Source: CAD feature listing. Evaluate the final solid. Frame: model axes, mm. Coordinates: 2 decimals unless noted, no trailing zeros. Write each loop counter-clockwise with the first axis right and the second up, starting at its lowest first coordinate (ties: lowest second). Pieces come first, ordered by that corner, then holes. Notation, with made-up numbers: (88, 87.25) -> (135, 87.25) arc R23 ccw to (135, 112.25) -> close; hole circle Ø4 at (65, -29.75). An arc over 180 degrees is marked (long way). Write item = value, one per line.
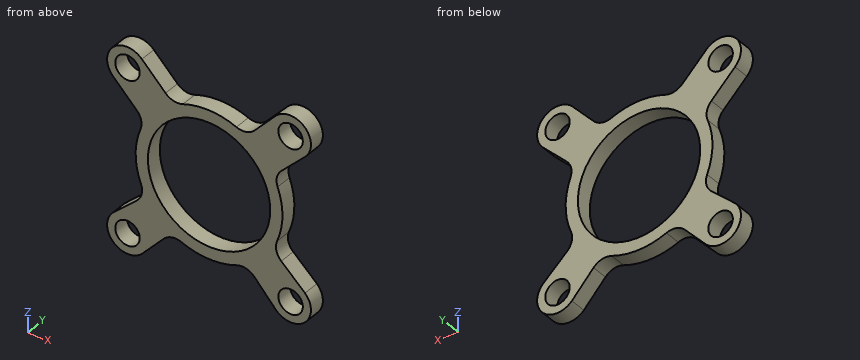
from build123d import *

# Parameters (mm, degrees)
SKETCH1_R           = 7.5
SKETCH1_R_2         = 1.5
BOSS_EXTRUDE1_DEPTH = 2
FILLET1_R           = 2


with BuildPart() as part:
    # Sketch1 → Boss-Extrude1 (new body)
    with BuildSketch(Plane(origin=(0, 0, 0), x_dir=(1, 0, 0), z_dir=(0, 1, 0))):
        with BuildLine():
            Line((-11.767766953, -8.232233047), (-7.881276583, -4.345742677))
            ThreePointArc((-7.881276583, -4.345742677), (-8.999066908, 0.129594703), (-7.75286903, 4.570888514))
            Line((-7.75286903, 4.570888514), (-11.767766953, 8.232233047))
            ThreePointArc((-11.767766953, 8.232233047), (-11.767766953, 11.767766953), (-8.232233047, 11.767766953))
            Line((-8.232233047, 11.767766953), (-4.570888514, 7.75286903))
            ThreePointArc((-4.570888514, 7.75286903), (0, 9), (4.570888514, 7.75286903))
            Line((4.570888514, 7.75286903), (8.232233047, 11.767766953))
            ThreePointArc((8.232233047, 11.767766953), (11.767766953, 11.767766953), (11.767766953, 8.232233047))
            Line((11.767766953, 8.232233047), (7.75286903, 4.570888514))
            ThreePointArc((7.75286903, 4.570888514), (8.999066908, 0.129594703), (7.881276583, -4.345742677))
            Line((7.881276583, -4.345742677), (11.767766953, -8.232233047))
            ThreePointArc((11.767766953, -8.232233047), (11.767766953, -11.767766953), (8.232233047, -11.767766953))
            Line((8.232233047, -11.767766953), (4.570888514, -7.75286903))
            ThreePointArc((4.570888514, -7.75286903), (0.129594703, -8.999066908), (-4.345742677, -7.881276583))
            Line((-4.345742677, -7.881276583), (-8.232233047, -11.767766953))
            ThreePointArc((-8.232233047, -11.767766953), (-11.767766953, -11.767766953), (-11.767766953, -8.232233047))
        make_face()
        Circle(SKETCH1_R, mode=Mode.SUBTRACT)
        with Locations((-10, -10)):
            Circle(SKETCH1_R_2, mode=Mode.SUBTRACT)
        with Locations((10, -10)):
            Circle(SKETCH1_R_2, mode=Mode.SUBTRACT)
        with Locations((10, 10)):
            Circle(SKETCH1_R_2, mode=Mode.SUBTRACT)
        with Locations((-10, 10)):
            Circle(SKETCH1_R_2, mode=Mode.SUBTRACT)
    extrude(amount=BOSS_EXTRUDE1_DEPTH)

    # Fillet1
    fillet1_edges = [part.edges().sort_by_distance(p)[0] for p in [
        (-7.881276583, 1, 4.345742677),
        (-7.75286903, 1, -4.570888514),
        (-4.570888514, 1, -7.75286903),
        (4.570888514, 1, -7.75286903),
        (7.75286903, 1, -4.570888514),
        (7.881276583, 1, 4.345742677),
        (4.570888514, 1, 7.75286903),
        (-4.345742677, 1, 7.881276583),
    ]]
    fillet(fillet1_edges, radius=FILLET1_R)


solid = part.part
1) Cut plane C-C, the plane y = 1.7. Give the number of separate pieces and of enclosed holes in the cut face, and give its area (3 significant figures).
Answer block:
separate_pieces = 1
enclosed_holes = 5
area = 193 mm2
2) Cut plane A-A, the plane x = 0. Output: boundary loops of the cut face in (y, z), and give its area (3 significant figures).
Answer block:
outline = (0, -9) -> (2, -9) -> (2, -7.5) -> (0, -7.5) -> close; (0, 7.5) -> (2, 7.5) -> (2, 9) -> (0, 9) -> close
area = 6.00 mm2
3) Cut plane D-D, the plane z = -10.5. Output: boundary loops of the cut face in (x, y), and give its area (3 significant figures).
Answer block:
outline = (-12.45, 0) -> (-11.41, 0) -> (-11.41, 2) -> (-12.45, 2) -> close; (-8.59, 0) -> (-7.08, 0) -> (-7.08, 2) -> (-8.59, 2) -> close; (7.08, 0) -> (8.59, 0) -> (8.59, 2) -> (7.08, 2) -> close; (11.41, 0) -> (12.45, 0) -> (12.45, 2) -> (11.41, 2) -> close
area = 10.2 mm2
4) Cut plane B-B, the plane z = 0. Output: boundary loops of the cut face in (x, y), and give its area (3 significant figures).
Answer block:
outline = (-9, 0) -> (-7.5, 0) -> (-7.5, 2) -> (-9, 2) -> close; (7.5, 0) -> (9, 0) -> (9, 2) -> (7.5, 2) -> close
area = 6.00 mm2
5) First-contact query: pin 1 Ø1 at (y, z) = (0.5, -8.5) entering from +X; pin 2 Ø5 at (x, z) = (-10, 10) entering from +Y; pin 3 Ø2.5 at (x, z) = (-10, -10) entering from +Y. Flat tips, straight axial feed; report the tip coordinate or a pass-through.
Answer block:
pin_1 = 12.29
pin_2 = 2
pin_3 = through
6) Material intervals for probe 1 along Z at (x, y) = (-10, 0.8); probe 2 along Z at (x, y) = (0.25, 0.1); probe 3 along X at (y, z) = (1.55, -10), sorted ascending. Write a range as [from, to].
Answer block:
probe_1 = [-12.5, -11.5], [-8.5, -6.62], [6.46, 8.5], [11.5, 12.5]
probe_2 = [-9, -7.5], [7.5, 9]
probe_3 = [-12.5, -11.5], [-8.5, -6.62], [6.62, 8.5], [11.5, 12.5]
